For this review, take the finished solid that the model builds, in its own axes (mm). Coordinates: 2 decimals unless noted, no trailing zeros. Order: outer loops, then holes, each group sorted by start corner. A loop starts at its lowest first (then second) coordinate and runs counter-clockwise, first axis right, second up.
from build123d import *

# Parameters (mm, degrees)
ESQUISSE1_W                = 2.54
ESQUISSE1_H                = 2.35
BOSS_EXTRU_1_DEPTH         = 2.5
BOSS_EXTRU_2_START         = -3
ESQUISSE2_R                = 0.325
BOSS_EXTRU_2_DEPTH         = 11.5
R_P_TITION_LIN_AIRE1_COUNT = 5
R_P_TITION_LIN_AIRE1_PITCH = 2.54


with BuildPart() as part:
    # Esquisse1 → Boss.-Extru.1 (new body)
    with BuildSketch(Plane(origin=(0, 0, 0), x_dir=(1, 0, 0), z_dir=(0, 1, 0))):
        with Locations((1.27, 1.175)):
            Rectangle(ESQUISSE1_W, ESQUISSE1_H)
    boss_extru_1 = extrude(amount=BOSS_EXTRU_1_DEPTH)

    # Esquisse2 → Boss.-Extru.2 (add)
    with BuildSketch(Plane(origin=(0, 0, 0), x_dir=(1, 0, 0), z_dir=(0, 1, 0)).offset(BOSS_EXTRU_2_START)):
        with Locations(Location((1.27, 1.175, 0), (0, 0, 270))):
            Circle(ESQUISSE2_R)
    boss_extru_2 = extrude(amount=BOSS_EXTRU_2_DEPTH)

    # Répétition linéaire1: Boss.-Extru.1, Boss.-Extru.2 ×5
    with Locations(*[(i * R_P_TITION_LIN_AIRE1_PITCH, 0, 0) for i in range(1, R_P_TITION_LIN_AIRE1_COUNT)]):
        add(boss_extru_1)
        add(boss_extru_2)


solid = part.part
1. The part is to be moulded in two halves that separate along X. For faces 1 (the face through (6, 1, -2.35)), 2 (the face through (0, 1, -1)), 3 (the face through (6, 2.5, -2)), say which applies: +X half, -X half, draft (parallel to the pull), parting line (faces both ways), or undercut.
Answer below:
face 1: draft
face 2: -X half
face 3: undercut
2. Take a section at D-D, the plane x = 10.25. Give the boundary of the cut face in (y, z), plus the area to 4 significant figures.
Answer below:
outline: (0, -2.35) - (2.5, -2.35) - (2.5, 0) - (0, 0) - close
area: 5.875 mm2
3. To check wall thickness, follow L1, parallel to Y at x = 8.5, z = -0.75; L2, parallel to Z at x = 1, y = 5.25; L3, parallel to Z at x = 11.5, y = 5.5. State the ranges of each line that lie inside material, in increasing order.
Answer below:
L1: y = 0 to 2.5
L2: z = -1.36 to -0.99
L3: z = -1.49 to -0.86
4. Take a section at C-C, the plane z = -2.05. Give the boundary of the cut face in (x, y).
Answer below:
outline: (0, 0) - (12.7, 0) - (12.7, 2.5) - (0, 2.5) - close
5. Take a section at A-A, the plane y = 6.5. Give the boundary of the cut face in (x, z) (3 decimals), plus the area to 3 significant figures.
Answer below:
outline: circle Ø0.65 at (1.27, -1.175); circle Ø0.65 at (3.81, -1.175); circle Ø0.65 at (6.35, -1.175); circle Ø0.65 at (8.89, -1.175); circle Ø0.65 at (11.43, -1.175)
area: 1.66 mm2
6. Clearance check with a flat-ended pin moving along its axis: pin 1 Ø4 at (x, y) = (9, 7.5) entering from -Z. State where the tip first meets the part, or that it passes through.
Answer below:
pin 1: stops at z = -1.5
7. Take a section at B-B, the plane x = 6.35. Give the boundary of the cut face in (y, z), plus the area to 3 significant figures.
Answer below:
outline: (-3, -1.5) - (0, -1.5) - (0, -2.35) - (2.5, -2.35) - (2.5, -1.5) - (8.5, -1.5) - (8.5, -0.85) - (2.5, -0.85) - (2.5, 0) - (0, 0) - (0, -0.85) - (-3, -0.85) - close
area: 11.7 mm2
